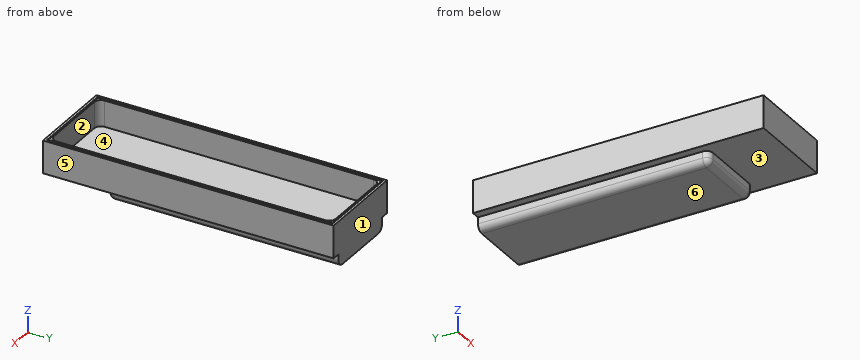
```python
from build123d import *

# Parameters (mm, degrees)
F0_W     = 70.739
F0_H     = 226.2886
F1_DEPTH = 25.4
F2_W     = 63.8302
F2_H     = 219.4306
F3_DEPTH = 20.32
F4_W     = 57.5818
F4_H     = 180.0606
F5_DEPTH = 10.16
F6_R     = 5.08
F7_W     = 66.8782
F7_H     = 222.4786
F7_W_2   = 65.3542
F7_H_2   = 220.9546
F8_DEPTH = 5


with BuildPart() as f1:
    # F0 (on Top) → F1 (new body)
    with BuildSketch(Plane.XY):
        with Locations((-23.397979, 9.605568)):
            Rectangle(F0_W, F0_H)
    extrude(amount=F1_DEPTH)

    # F2 (on face) → F3 (cut)
    with BuildSketch(Plane.XY.offset(25.4)):
        with Locations((-23.397979, 9.605568)):
            Rectangle(F2_W, F2_H)
    extrude(amount=-F3_DEPTH, mode=Mode.SUBTRACT)

    # F4 (on face) → F5 (join)
    with BuildSketch(Plane(origin=(0, 0, 0), x_dir=(1, 0, 0), z_dir=(0, 0, -1))):
        with Locations((-23.397979, -32.719568)):
            Rectangle(F4_W, F4_H)
    extrude(amount=F5_DEPTH)

    # F6
    f6_edges = [f1.edges().sort_by_distance(p)[0] for p in [
        (-23.397979, -57.310732, -10.16),
        (5.392921, 32.719568, -10.16),
        (-52.188879, 32.719568, -10.16),
        (5.392921, -57.310732, -5.08),
        (-52.188879, -57.310732, -5.08),
        (8.517121, -100.109732, 15.24),
        (8.517121, 119.320868, 15.24),
        (-55.313079, 119.320868, 15.24),
        (-55.313079, -100.109732, 15.24),
    ]]
    fillet(f6_edges, radius=F6_R)

    # F7 (on face) → F8 (cut)
    with BuildSketch(Plane.XY.offset(25.4)):
        with Locations((-23.397979, 9.605568)):
            Rectangle(F7_W, F7_H)
        with Locations((-23.397979, 9.605568)):
            Rectangle(F7_W_2, F7_H_2, mode=Mode.SUBTRACT)
    extrude(amount=-F8_DEPTH, mode=Mode.SUBTRACT)


solid = f1.part
```
Verification items for the finished model (mm, model axes). Face numbers are marked on the shaded views. A direction names the side the tool comes from. Round coordinates to 2 decimals unless told otherwise and drop trailing zeros. Write each loop counter-clockwise with the first axis right and the second up, starting at its lowest first coordinate (ties: lowest second). Pieces come first, ordered by that corner, then holes.
1. Section check A-A on x = -30.5. Enter the section's corners in (y, z), plus the area to 3 significant figures.
2. Section check C-C on y = -28.5. Enter the section's corners in (x, z), plus the area to 3 significant figures.
3. Scan lines: L1, parallel to Y at x = -50.5, z = 23; L2, parallel to X at y = 24.5, z = 24.5; L3, parallel to Y at x = -24.5, z = 13.5. Record each from-to range of solid material in increasing order.
4. Draft check along X on the marked faces 4, 5 and 6. Enter one of: +X half, -X half, draft (parallel to the pull), parting line (faces both ways), or undercut.
5. Access from +Z, -Z, +X, -X, +Y, -Y to the whole of each face (thin tool, end or side, straight path). Record for the marked faces 1, 2 and 3.
6. Section check B-B on z = 15. Enter the section's corners in (x, y).
7. Gauge pin test, flat ends, axial feed: P1, Ø1.5, axis at x = -34.5, z = -2.5, coming from the -Y side; P2, Ø20, axis at x = -15, y = -20, coming from the +Z side. Record the tip position at first contact, or that the pin passes through.
Answer:
1. outline: (-103.54, 0) - (-57.31, 0) - (-57.31, -5.08) arc R5.08 ccw to (-52.23, -10.16) - (122.75, -10.16) - (122.75, 25.4) - (120.84, 25.4) - (120.84, 20.4) - (120.08, 20.4) - (120.08, 25.4) - (119.32, 25.4) - (119.32, 5.08) - (-100.11, 5.08) - (-100.11, 25.4) - (-100.87, 25.4) - (-100.87, 20.4) - (-101.63, 20.4) - (-101.63, 25.4) - (-103.54, 25.4) - close
1. area: 3,110 mm2
2. outline: (-58.77, 0) - (-52.19, 0) - (-52.19, -5.08) arc R5.08 ccw to (-47.11, -10.16) - (0.31, -10.16) arc R5.08 ccw to (5.39, -5.08) - (5.39, 0) - (11.97, 0) - (11.97, 25.4) - (10.04, 25.4) - (10.04, 20.4) - (9.28, 20.4) - (9.28, 25.4) - (8.52, 25.4) - (8.52, 5.08) - (-55.31, 5.08) - (-55.31, 25.4) - (-56.08, 25.4) - (-56.08, 20.4) - (-56.84, 20.4) - (-56.84, 25.4) - (-58.77, 25.4) - close
2. area: 1,070 mm2
3. L1: y = -103.54 to -101.63, -100.87 to -100.1, 119.31 to 120.08, 120.84 to 122.75
3. L2: x = -58.77 to -56.84, -56.08 to -55.31, 8.52 to 9.28, 10.04 to 11.97
3. L3: y = -103.54 to -100.11, 119.32 to 122.75
4. face 4: undercut
4. face 5: +X half
4. face 6: draft
5. face 1: +Z, -Z, +X, -X, +Y
5. face 2: +Z
5. face 3: -Z, -Y
6. outline: (-58.77, -103.54) - (11.97, -103.54) - (11.97, 122.75) - (-58.77, 122.75) - close; hole (-55.31, -95.03) arc R5.08 ccw to (-50.23, -100.11) - (3.44, -100.11) arc R5.08 ccw to (8.52, -95.03) - (8.52, 114.24) arc R5.08 ccw to (3.44, 119.32) - (-50.23, 119.32) arc R5.08 ccw to (-55.31, 114.24) - close
7. P1: stops at y = -57.31
7. P2: stops at z = 5.08
